```python
from build123d import *

# Parameters (mm, degrees)
AUFSATZ_LINEAR_AUSTRAGEN3_DEPTH = 20
AUFSATZ_LINEAR_AUSTRAGEN4_DEPTH = 2
SKIZZE3_R                       = 6.5
AUFSATZ_LINEAR_AUSTRAGEN5_DEPTH = 1.2
SCHNITT_LINEAR_AUSTRAGEN1_REACH = 53.652
SKIZZE4_R                       = 2
SKIZZE6_W                       = 7
SKIZZE6_H                       = 4
AUFSATZ_LINEAR_AUSTRAGEN6_DEPTH = 4
SKIZZE7_R                       = 4.5
AUFSATZ_LINEAR_AUSTRAGEN7_DEPTH = 0.5
SKIZZE8_R                       = 3
AUFSATZ_LINEAR_AUSTRAGEN8_DEPTH = 4
VERRUNDUNG3_R                   = 2


with BuildPart() as part:
    # Skizze1 → Aufsatz-Linear austragen3 (new body)
    with BuildSketch(Plane(origin=(0, 0, 0), x_dir=(0, 0, -1), z_dir=(1, 0, 0))):
        Polygon((-11.014679398, 22.752092755), (-11.014679398, 28.752092755), (29.985320602, 28.752092755), (29.985320602, 22.752092755), (36.985320602, 22.752092755), (36.985320602, 20.152092755), (29.985320602, 20.152092755), (29.985320602, -7.247907245), (-11.014679398, -7.247907245), (-11.014679398, 20.152092755), (-18.014679398, 20.152092755), (-18.014679398, 22.752092755), align=None)
    extrude(amount=AUFSATZ_LINEAR_AUSTRAGEN3_DEPTH)

    # Skizze2 → Aufsatz-Linear austragen4 (add)
    with BuildSketch(Plane(origin=(0, 28.752092755, 0), x_dir=(1, 0, 0), z_dir=(0, 1, 0))):
        with BuildLine():
            Line((0, -1.014679398), (0, 23.985320602))
            Line((0, 23.985320602), (6.258342613, 23.985320602))
            ThreePointArc((6.258342613, 23.985320602), (10, 25.985320602), (13.741657387, 23.985320602))
            Line((13.741657387, 23.985320602), (20, 23.985320602))
            Line((20, 23.985320602), (20, -1.014679398))
            ThreePointArc((20, -1.014679398), (10, -11.014679398), (0, -1.014679398))
        make_face()
    extrude(amount=AUFSATZ_LINEAR_AUSTRAGEN4_DEPTH)

    # Skizze3 → Aufsatz-Linear austragen5 (add)
    with BuildSketch(Plane(origin=(0, 30.752092755, 0), x_dir=(1, 0, 0), z_dir=(0, 1, 0))):
        with Locations(Location((10, -2.014679398, 0), (0, 0, 270))):
            Circle(SKIZZE3_R)
    extrude(amount=AUFSATZ_LINEAR_AUSTRAGEN5_DEPTH)

    # Skizze4 → Schnitt-Linear austragen1 (cut, up to next)
    with BuildSketch(Plane(origin=(0, 22.752092755, 0), x_dir=(1, 0, 0), z_dir=(0, 1, 0)), mode=Mode.PRIVATE) as schnitt_linear_austragen1_sk1:
        with Locations(Location((5.25, -14.514679398, 0), (0, 0, 270))):
            Circle(SKIZZE4_R)
    schnitt_linear_austragen1_tool1 = extrude(schnitt_linear_austragen1_sk1.sketch, amount=-SCHNITT_LINEAR_AUSTRAGEN1_REACH, mode=Mode.PRIVATE) & part.part
    # Skizze4 → Schnitt-Linear austragen1 (cut, up to next)
    with BuildSketch(Plane(origin=(0, 22.752092755, 0), x_dir=(1, 0, 0), z_dir=(0, 1, 0)), mode=Mode.PRIVATE) as schnitt_linear_austragen1_sk2:
        with Locations(Location((14.75, -14.514679398, 0), (0, 0, 270))):
            Circle(SKIZZE4_R)
    schnitt_linear_austragen1_tool2 = extrude(schnitt_linear_austragen1_sk2.sketch, amount=-SCHNITT_LINEAR_AUSTRAGEN1_REACH, mode=Mode.PRIVATE) & part.part
    # Skizze4 → Schnitt-Linear austragen1 (cut, up to next)
    with BuildSketch(Plane(origin=(0, 22.752092755, 0), x_dir=(1, 0, 0), z_dir=(0, 1, 0)), mode=Mode.PRIVATE) as schnitt_linear_austragen1_sk3:
        with Locations(Location((14.75, 33.485320602, 0), (0, 0, 270))):
            Circle(SKIZZE4_R)
    schnitt_linear_austragen1_tool3 = extrude(schnitt_linear_austragen1_sk3.sketch, amount=-SCHNITT_LINEAR_AUSTRAGEN1_REACH, mode=Mode.PRIVATE) & part.part
    # Skizze4 → Schnitt-Linear austragen1 (cut, up to next)
    with BuildSketch(Plane(origin=(0, 22.752092755, 0), x_dir=(1, 0, 0), z_dir=(0, 1, 0)), mode=Mode.PRIVATE) as schnitt_linear_austragen1_sk4:
        with Locations(Location((5.25, 33.485320602, 0), (0, 0, 270))):
            Circle(SKIZZE4_R)
    schnitt_linear_austragen1_tool4 = extrude(schnitt_linear_austragen1_sk4.sketch, amount=-SCHNITT_LINEAR_AUSTRAGEN1_REACH, mode=Mode.PRIVATE) & part.part
    add(schnitt_linear_austragen1_tool1.solids().sort_by_distance((5.25, 22.752093, 14.514679))[0], mode=Mode.SUBTRACT)
    add(schnitt_linear_austragen1_tool2.solids().sort_by_distance((14.75, 22.752093, 14.514679))[0], mode=Mode.SUBTRACT)
    add(schnitt_linear_austragen1_tool3.solids().sort_by_distance((14.75, 22.752093, -33.485321))[0], mode=Mode.SUBTRACT)
    add(schnitt_linear_austragen1_tool4.solids().sort_by_distance((5.25, 22.752093, -33.485321))[0], mode=Mode.SUBTRACT)

    # Skizze6 → Aufsatz-Linear austragen6 (add)
    with BuildSketch(Plane.XY.offset(11.014679398)):
        with Locations((10, -1.747907245)):
            Rectangle(SKIZZE6_W, SKIZZE6_H)
    extrude(amount=AUFSATZ_LINEAR_AUSTRAGEN6_DEPTH)

    # Skizze7 → Aufsatz-Linear austragen7 (add)
    with BuildSketch(Plane(origin=(0, 31.952092755, 0), x_dir=(1, 0, 0), z_dir=(0, 1, 0))):
        with Locations(Location((10, -2.014679398, 0), (0, 0, 270))):
            Circle(SKIZZE7_R)
    extrude(amount=AUFSATZ_LINEAR_AUSTRAGEN7_DEPTH)

    # Skizze8 → Aufsatz-Linear austragen8 (add)
    with BuildSketch(Plane(origin=(0, 32.452092755, 0), x_dir=(1, 0, 0), z_dir=(0, 1, 0))):
        with Locations(Location((10, -2.014679398, 0), (0, 0, 270))):
            Circle(SKIZZE8_R)
    extrude(amount=AUFSATZ_LINEAR_AUSTRAGEN8_DEPTH)

    # Verrundung3
    verrundung3_edges = [part.edges().sort_by_distance(p)[0] for p in [
        (0, 21.452092755, 18.014679398),
        (0, 21.452092755, -36.985320602),
        (20, 21.452092755, -36.985320602),
        (20, 21.452092755, 18.014679398),
    ]]
    fillet(verrundung3_edges, radius=VERRUNDUNG3_R)


solid = part.part
```
For this review, take the finished solid that the model builds, in its own axes (mm). A direction names the side the tool comes from. Give positions to 0.01 mm unless a question says otherwise; leave off trailing zeros. Order: outer loops, then holes, each group sorted by start corner. A loop starts at its lowest first (then second) coordinate and runs counter-clockwise, first axis right, second up.
1) Insertion check: pin 1 (6.5 mm diameter, centred on x = 5.25, z = -33.49, fed in from +Y); pin 2 (6 mm diameter, centred on x = 7.5, y = 12, fed in from +Z); pin 3 (6.5 mm diameter, centred on x = 14.75, z = -33.49, fed in from -Y). Each pin has a flat end and moves straight along its axis. Give the tip position at first contact, or say it passes through.
2) Take a section at A-A (x = 4.25). Give the boundary of the cut face in (y, z).
3) The part is to be moulded in two halves that separate along Z. For faces 1 (the face through (16.733, 21.47, 14.254)), 2 (the face through (5.851, 21.47, -31.578)), 3 (the face through (6.5, -2, 13)), 4 (the face through (19.399, 21.434, -36.415)), say which applies: released by +Z, released by -Z, zero draft, split by the parting line, or undercut.
4) Take a section at D-D (z = -11). Give the boundary of the cut face in (x, y), then the cut area to 3 significant figures.
5) Wall thickness on line 1 (Z direction, x = 5, y = 20.5); line 2 (Z direction, x = 2.5, y = 11.5); line 3 (Y direction, x = 18.75, z = 2): over which ranges is each line inside the solid? List them lowest first.
6) Take a section at C-C (z = 2.5). Give the boundary of the cut face in (x, y), then the cut area to 3 significant figures.
7) Take a section at B-B (y = 23.5). Give the boundary of the cut face in (x, z), then the cut area to 3 significant figures.
8) For faces 5 (the face through (6.6, 21.47, 13.04)), 6 (the face through (13.5, -2, 13)), 7 (the face through (10, 20.152, 14)), 8 (the face through (10, -2, 15.015)), list the 3-axis set-ups (+Z, -Z, +X, -X, +Y, -Y) from which the entire face can be reached by the end or side of a thin tool; tool diameter is ignored.
Derived:
1. pin 1: stops at y = 22.75
1. pin 2: stops at z = 11.01
1. pin 3: stops at y = 20.15
2. outline: (-7.25, -29.99) - (20.15, -29.99) - (20.15, -31.75) - (22.75, -31.75) - (22.75, -29.99) - (28.75, -29.99) - (28.75, -23.99) - (30.75, -23.99) - (30.75, -1.02) - (31.95, -1.02) - (31.95, 5.05) - (30.75, 5.05) - (30.75, 9.2) - (28.75, 9.2) - (28.75, 11.01) - (22.75, 11.01) - (22.75, 12.78) - (20.15, 12.78) - (20.15, 11.01) - (-7.25, 11.01) - close; (20.15, -36.99) - (22.75, -36.99) - (22.75, -35.22) - (20.15, -35.22) - close; (20.15, 16.25) - (22.75, 16.25) - (22.75, 18.01) - (20.15, 18.01) - close
3. face 1: undercut
3. face 2: undercut
3. face 3: zero draft
3. face 4: released by -Z
4. outline: (0, -7.25) - (20, -7.25) - (20, 30.75) - (0, 30.75) - close
4. area: 760 mm2
5. line 1: z = -36.99 to -35.47, -31.5 to 12.53, 16.5 to 18.01
5. line 2: z = -29.99 to 11.01
5. line 3: y = -7.25 to 30.75
6. outline: (0, -7.25) - (20, -7.25) - (20, 28.75) - (19.89, 28.75) - (19.89, 30.75) - (16.48, 30.75) - (16.48, 31.95) - (14.47, 31.95) - (14.47, 32.45) - (12.96, 32.45) - (12.96, 36.45) - (7.04, 36.45) - (7.04, 32.45) - (5.53, 32.45) - (5.53, 31.95) - (3.52, 31.95) - (3.52, 30.75) - (0.11, 30.75) - (0.11, 28.75) - (0, 28.75) - close
6. area: 803 mm2
7. outline: (0, -29.99) - (20, -29.99) - (20, 11.01) - (0, 11.01) - close
7. area: 820 mm2
8. face 5: +Y
8. face 6: +Z, +X, -Y
8. face 7: +Z, +X, -X
8. face 8: +Z, +X, -X, -Y
